Read the model definition and answer for the solid it produces. Units are mm, in the model's axes. Coordinates: 2 decimals unless noted, no trailing zeros. Write each loop counter-clockwise with the first axis right and the second up, starting at its lowest first coordinate (ties: lowest second). Pieces come first, ordered by that corner, then holes.
(1) Section A-A on x = -79.5 is taken. Write down the section's boundary in (y, z).
(2) Given pin 1 (1 mm diameter, centred on x = 87.5, z = -55.5, fed in from -Y), flat-ended and moving along its own axis, determine where the tip first touches the part or whether it passes through.
(3) Find the intervals of material crossed by probe 1 along Z at (x, y) = (93.5, 4.6); probe 2 along X at (y, z) = (2.5, 14.5); probe 3 along Z at (x, y) = (73, 3.5), in increasing order.
(4) Section B-B on y = 0.9 is taken. State how many separate pieces and enclosed holes the cut face has, then the cut area to 3 significant figures.
Autodesk Inventor part; units mm, degrees
ref_plane "YZ Plane" through (0, 0, 0) normal (1, 0, 0) x (0, 1, 0)
ref_plane "XZ Plane" through (0, 0, 0) normal (0, 1, 0) x (-1, 0, 0)
ref_plane "XY Plane" through (0, 0, 0) normal (0, 0, 1) x (1, 0, 0)
sketch "Esquisse1" plane through (0, 0, 0) normal (0, 1, 0) x (-1, 0, 0)
  line L0 (98.2051, 94.359) -> (-201.7949, 94.359)
  line L1 (-201.7949, 94.359) -> (-201.7949, -105.641)
  line L2 (-201.7949, -105.641) -> (98.2051, -105.641)
  line L3 (98.2051, -105.641) -> (98.2051, 94.359)
  point P0 (0, 0)
  dimension "d0" = 200
  dimension "d1" = 300
extrude "Extrusion1" add sketch "Esquisse1" along normal blind 5
sketch "Esquisse2" plane through (0, 5, 0) normal (0, 1, 0) x (1, 0, 0)
  line L0 (89.9575, -12.359) -> (-80.036, -12.359)
  line L1 (89.9575, -7.359) -> (-80.036, -7.359)
  line L2 (-80.036, -12.359) -> (-80.036, -7.359)
  line L3 (89.9575, -12.359) -> (89.9575, -7.359)
  line L4 (-90.036, -22.359) -> (99.9575, -22.359)
  line L5 (99.9575, -22.359) -> (99.9575, 2.641)
  line L6 (99.9575, 2.641) -> (-90.036, 2.641)
  line L7 (-90.036, 2.641) -> (-90.036, -22.359)
  point P0 (0, 0)
  dimension "d4" = 10
  dimension "d5" = 10
  dimension "d6" = 10
  dimension "d7" = 10
extrude "Extrusion2" cut sketch "Esquisse2" against normal through all contours L0 L2 L1 L3 | L7 L6 L5 L4
sketch "Esquisse3" plane through (0, 0, 0) normal (0, -1, 0) x (1, 0, 0)
  circle A0 centre (56.2949, 33.359) radius 1
  line L0 (57.2949, 15.359) -> (55.2949, 15.359)
  circle A1 centre (56.2949, 41.359) radius 1
  circle A2 centre (64.2949, 41.359) radius 1
  circle A3 centre (72.2949, 33.359) radius 1
  circle A4 centre (72.2949, 41.359) radius 1
  circle A5 centre (72.2949, 25.359) radius 1
  circle A6 centre (64.2949, 25.359) radius 1
  circle A7 centre (56.2949, 25.359) radius 1
  point P0 (0, 0)
extrude "Extrusion3" cut sketch "Esquisse3" against normal through all
properties part number "face-lateral"
Response:
1. outline: (0, -105.64) - (5, -105.64) - (5, -2.64) - (0, -2.64) - close; (0, 22.36) - (5, 22.36) - (5, 94.36) - (0, 94.36) - close
2. pin 1: stops at y = 0
3. probe 1: z = -105.64 to -2.64, 22.36 to 94.36
3. probe 2: x = -98.21 to -90.04, 99.96 to 201.79
3. probe 3: z = -105.64 to -2.64, 22.36 to 24.65, 26.07 to 32.65, 34.07 to 40.65, 42.07 to 94.36
4. separate pieces: 1
4. enclosed holes: 9
4. area: 55,200 mm2
